```python
from build123d import *

# Parameters (mm, degrees)
F0_W     = 12.7
F0_H     = 50.8
F0_W_2   = 3.175
F0_H_2   = 3.175
F1_DEPTH = 6.35
F2_DEPTH = 3.175


with BuildPart() as f1:
    # F0 (on Front) → F1 (new body, symmetric)
    with BuildSketch(Plane.XZ):
        Polygon((0, 13.925004), (12.7, 13.925004), (-21.420162, 48.045166), (-21.420162, 45.339696), (-21.420162, 40.685079), (-21.420162, 35.345166), align=None)
        with Locations((6.35, -11.474996)):
            Rectangle(F0_W, F0_H)
        with Locations((5.976701, -31.348965)):
            Rectangle(F0_W_2, F0_H_2, mode=Mode.SUBTRACT)
    extrude(amount=F1_DEPTH, both=True)

    # F0 (on Front) → F2 (join, symmetric)
    with BuildSketch(Plane.XZ):
        Polygon((-21.420162, 40.685079), (-21.420162, 45.339696), (-56.897912, 28.29555), (-55.081078, 24.513772), align=None)
    extrude(amount=F2_DEPTH, both=True)


solid = f1.part
```
Design review of the part built by this model. Coordinates are the model's own, in mm. A direction names the side the tool comes from. Round coordinates to 2 decimals unless told otherwise and drop trailing zeros. Order: outer loops, then holes, each group sorted by start corner. A loop starts at its lowest first (then second) coordinate and runs counter-clockwise, first axis right, second up. Notation, with made-up numbers: (-28.5, -36) - (-1.5, -36) arc R23 ccw to (-1.5, -14) - close; hole circle Ø2 at (81.5, 61). An arc over 180 degrees is marked (long way). One line per question, with ' | ' between items.
Item 1: Draft analysis for pull direction X (two halves, no side actions). For faces 6 (the face through (12.7, 0, -12)), 7 (the face through (6, 0, -36.875)), 8 (the face through (-56, -0.04, 26.43)), 9 (the face through (-38.486, -0.044, 32.486)), state which applies: +X half, -X half, draft (parallel to the pull), parting line (faces both ways), or undercut.
Checks:
face 6: +X half | face 7: draft | face 8: -X half | face 9: undercut
Item 2: Take a section at B-B, the plane z = 37.5. Write out the cut boundary in (x, y) (3 decimals), then the cut area to 3 significant figures.
Checks:
outline: (-37.739, -3.175) - (-28.05, -3.175) - (-28.05, 3.175) - (-37.739, 3.175) - close; (-21.42, -6.35) - (-10.875, -6.35) - (-10.875, 6.35) - (-21.42, 6.35) - close | area: 195 mm²
Item 3: Take a section at C-C, the plane z = -20. Write out the cut boundary in (x, y), then the cut area to 3 significant figures.
Checks:
outline: (0, -6.35) - (12.7, -6.35) - (12.7, 6.35) - (0, 6.35) - close | area: 161 mm²
Item 4: For P1, Ø3.5, axis at x = 6.5, y = -1, coming from the +Z side (3 decimals); P2, Ø5, axis at x = -10, y = -4.5, coming from the -Z side (3 decimals); P3, Ø2.5, axis at y = -0.5, z = -30.5, coming from the -X side, all flat-tipped, find the tip position at first contact; note any pin that passes through.
Checks:
P1: z = 21.875 | P2: z = 21.425 | P3: x = 0
Item 5: Wall thickness on line 1 (X direction, y = -1, z = 8.5); line 2 (Y direction, x = -45, z = 31.5) (3 decimals); line 3 (X direction, y = -2.75, z = 34.5) (3 decimals): over which ranges is each line inside the solid? List them lowest first. Write a range as [from, to].
Checks:
line 1: [0, 12.7] | line 2: [-3.175, 3.175] | line 3: [-43.983, -34.295], [-20.575, -7.875]
Item 6: Take a section at A-A, the plane y = -2. Write out the cut boundary in (x, z) (3 decimals).
Checks:
outline: (-56.898, 28.296) - (-55.081, 24.514) - (-21.42, 40.685) - (-21.42, 35.345) - (0, 13.925) - (0, -36.875) - (12.7, -36.875) - (12.7, 13.925) - (-21.42, 48.045) - (-21.42, 45.34) - close; hole (4.389, -32.936) - (7.564, -32.936) - (7.564, -29.761) - (4.389, -29.761) - close
Item 7: Take a section at D-D, the plane x = -5. Write out the cut boundary in (y, z) (3 decimals), then the cut area to 3 significant figures.
Checks:
outline: (-6.35, 18.925) - (6.35, 18.925) - (6.35, 31.625) - (-6.35, 31.625) - close | area: 161 mm²
Item 8: Machinability: for faces 1 (the face through (0, 0, -12)), 2 (the face through (-39, -3.175, 35)), 3 (the face through (-39, 3.175, 35)), 4 (the face through (7.564, 0, -31)), 5 (the face through (-10.86, -0.089, 24.785)), which of the approach directions +Z, -Z, +X, -X, +Y, -Y give a long, thin tool a straight path to every point of the face, cutting with its end or side? Answer none if there is none.
Checks:
face 1: -Z, -X, +Y, -Y | face 2: +Z, -Z, -X, -Y | face 3: +Z, -Z, -X, +Y | face 4: +Y, -Y | face 5: -Z, +Y, -Y
